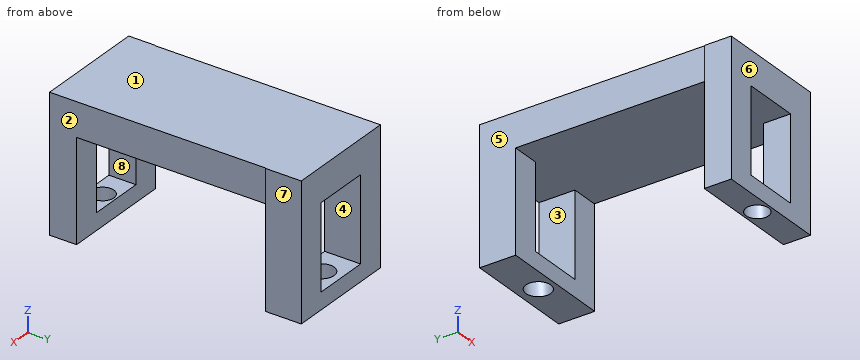
```python
from build123d import *

# Parameters (mm, degrees)
SZKIC2_W                      = 10
SZKIC2_H                      = 3.2
SZKIC2_R                      = 1.10000034
DODANIE_WYCI_GNI_CIE1_DEPTH   = 12
SZKIC2_H_2                    = 2.4000007
SZKIC2_R_2                    = 1.00000054
DODANIE_WYCI_GNI_CIE1_2_DEPTH = 12
SZKIC3_W                      = 5
SZKIC3_H                      = 3.2
SZKIC3_H_2                    = 2.4000007
WYTNIJ_WYCI_GNI_CIE1_DEPTH    = 10.5
SZKIC4_W                      = 9.95021092
SZKIC4_H                      = 22.39976104
DODANIE_WYCI_GNI_CIE2_DEPTH   = 3


with BuildPart() as part:
    # Szkic2 → Dodanie-wyci_gni_cie1 (new body)
    with BuildSketch(Plane.XY.offset(158.832884642)):
        with Locations((-14.923531216, -1.67449554)):
            Rectangle(SZKIC2_W, SZKIC2_H)
        with Locations((-14.923531216, -1.77449554)):
            Circle(SZKIC2_R, mode=Mode.SUBTRACT)
    extrude(amount=DODANIE_WYCI_GNI_CIE1_DEPTH)


with BuildPart() as body_2:
    # Szkic2 → Dodanie-wyci_gni_cie1 2 (new body)
    with BuildSketch(Plane.XY.offset(158.832884642)):
        with Locations((-14.973320296, -21.27425623)):
            Rectangle(SZKIC2_W, SZKIC2_H_2)
        with Locations((-14.973320296, -21.27425588)):
            Circle(SZKIC2_R_2, mode=Mode.SUBTRACT)
    extrude(amount=DODANIE_WYCI_GNI_CIE1_2_DEPTH)


with BuildPart() as wytnij_wyci_gni_cie1_tool:
    # Szkic3 → Wytnij-wyci_gni_cie1 (new body)
    with BuildSketch(Plane.XY.offset(170.832884642)):
        with Locations((-14.923531216, -1.67449554)):
            Rectangle(SZKIC3_W, SZKIC3_H)
        with Locations((-14.973320296, -21.27425623)):
            Rectangle(SZKIC3_W, SZKIC3_H_2)
    extrude(amount=-WYTNIJ_WYCI_GNI_CIE1_DEPTH)


with BuildPart() as part_1:
    add(part.part)

    # Wytnij-wyci_gni_cie1: cut by wytnij_wyci_gni_cie1_tool
    add(wytnij_wyci_gni_cie1_tool.part, mode=Mode.SUBTRACT)



with BuildPart() as body_2_1:
    add(body_2.part)

    # Wytnij-wyci_gni_cie1: cut by wytnij_wyci_gni_cie1_tool
    add(wytnij_wyci_gni_cie1_tool.part, mode=Mode.SUBTRACT)


with BuildPart() as part_2:
    add(part_1.part)

    add(body_2_1.part)  # Dodanie-wyci_gni_cie2 merges body 2
    # Szkic4 → Dodanie-wyci_gni_cie2 (add)
    with BuildSketch(Plane.XY.offset(170.832884642)):
        with Locations((-14.948425756, -11.27437606)):
            Rectangle(SZKIC4_W, SZKIC4_H)
    extrude(amount=-DODANIE_WYCI_GNI_CIE2_DEPTH)


solid = part_2.part
```
Geometry: final body of the model. Coordinates: model frame, mm. Face numbers are marked on the shaded views. A direction names the side the tool comes from. Give positions to 0.01 mm unless a question says otherwise; leave off trailing zeros. Order: outer loops, then holes, each group sorted by start corner. A loop starts at its lowest first (then second) coordinate and runs counter-clockwise, first axis right, second up. Notation, with made-up numbers: (-14.75, 51.25) -> (25.25, 51.25) arc R17 cw to (25.25, 78.25) -> close; hole circle Ø11 at (18.25, 82.25). An arc over 180 degrees is marked (long way). Write each question's results on one line, items separated by ' | '. Start each with the question number.
1) Draft query along X for the marked faces 6, 7 and 8. Return one class per face: pulls with the +X half, pulls with the -X half, needs draft (parallel to the pull), parting line crosses it, or undercut.
2) Section C-C (x = -11.5). Return loops of the section in (y, z), then the cut area to 3 significant figures.
3) Section D-D (y = -2.5). Return loops of the section in (x, z), then the cut area to 3 significant figures.
4) First-contact query: pin 1 (6 mm diameter, centred on y = -5, z = 162.5, fed in from -X); pin 2 (3.5 mm diameter, centred on y = -9.5, z = 167.5, fed in from +X); pin 3 (5 mm diameter, centred on x = -14, y = -7.5, fed in from -Z). Flat tips, straight axial feed; report the tip coordinate or a pass-through.
5) Section A-A (x = -16.5). Return loops of the section in (y, z).
6) Line query: line 1 (Y direction, x = -18.25, z = 160.25); line 2 (Y direction, x = -15.75, z = 160); line 3 (X direction, y = -2, z = 167.5). Output: solid intervals per line, ascending. Write a range as from..to.
7) Set-up query: the marked faces 1, 2, 3, 4 and 5. Return all of +Z, -Z, +X, -X, +Y, -Y with unobstructed straight access to the full face (end or side cutting, diameter ignored); none if empty.
8) Section B-B (z = 162.5). Return loops of the section in (x, y), then the cut area to 3 significant figures.
Calculated:
1) face 6: needs draft | face 7: pulls with the +X half | face 8: undercut
2) outline: (-22.47, 158.83) -> (-20.07, 158.83) -> (-20.07, 167.83) -> (-3.27, 167.83) -> (-3.27, 158.83) -> (-0.07, 158.83) -> (-0.07, 170.83) -> (-22.47, 170.83) -> close | area: 118 mm2
3) outline: (-19.92, 158.83) -> (-15.75, 158.83) -> (-15.75, 160.33) -> (-17.42, 160.33) -> (-17.42, 167.83) -> (-12.42, 167.83) -> (-12.42, 160.33) -> (-14.1, 160.33) -> (-14.1, 158.83) -> (-9.92, 158.83) -> (-9.92, 170.83) -> (-19.92, 170.83) -> close | area: 80.0 mm2
4) pin 1: x = -19.92 | pin 2: x = -9.97 | pin 3: z = 167.83
5) outline: (-22.47, 158.83) -> (-20.07, 158.83) -> (-20.07, 160.33) -> (-22.47, 160.33) -> close; (-22.47, 167.83) -> (-0.07, 167.83) -> (-0.07, 170.83) -> (-22.47, 170.83) -> close; (-3.27, 158.83) -> (-0.07, 158.83) -> (-0.07, 160.33) -> (-3.27, 160.33) -> close
6) line 1: -22.47..-20.07, -3.27..-0.07 | line 2: -22.47..-21.9, -20.64..-20.07, -3.27..-2.5, -1.05..-0.07 | line 3: -19.92..-17.42, -12.42..-9.92
7) face 1: +Z, +X, -X, +Y, -Y | face 2: +Z, -Z, +X, -Y | face 3: +Y | face 4: +Y, -Y | face 5: +Z, -Z, -X, +Y
8) outline: (-19.97, -22.47) -> (-17.47, -22.47) -> (-17.47, -20.07) -> (-19.97, -20.07) -> close; (-19.92, -3.27) -> (-17.42, -3.27) -> (-17.42, -0.07) -> (-19.92, -0.07) -> close; (-12.47, -22.47) -> (-9.97, -22.47) -> (-9.97, -20.07) -> (-12.47, -20.07) -> close; (-12.42, -3.27) -> (-9.92, -3.27) -> (-9.92, -0.07) -> (-12.42, -0.07) -> close | area: 28.0 mm2
